Geometry: final body of the model. Coordinates: model frame, mm. A direction names the side the tool comes from. Give positions to 0.01 mm unless a question says otherwise; leave off trailing zeros. Order: outer loops, then holes, each group sorted by start corner. A loop starts at its lowest first (then second) coordinate and runs counter-clockwise, first axis right, second up. Notation, with made-up numbers: (64.25, 55.25) -> (104.25, 55.25) arc R13 ccw to (104.25, 61.25) -> close; hole circle Ø5 at (-35, 81). An arc over 180 degrees is marked (long way). One line per question, with ' | ' between items.
from build123d import *

# Parameters (mm, degrees)
F1_DEPTH = 6.35
F3_DEPTH = 1.27
F5_DEPTH = 18.542


with BuildPart() as f1:
    # F0 (on Top) → F1 (new body)
    with BuildSketch(Plane.XY):
        with BuildLine():
            Line((8.6645979291, 6.620054795), (2.0859979291, 6.620054795))
            ThreePointArc((2.0859979291, 6.620054795), (-1.2007758112, 5.2586285353), (-2.5622020709, 1.971854795))
            Line((-2.5622020709, 1.971854795), (-2.5622020709, -4.606745205))
            ThreePointArc((-2.5622020709, -4.606745205), (-1.2007758112, -7.8935189453), (2.0859979291, -9.254945205))
            Line((2.0859979291, -9.254945205), (8.6645979291, -9.254945205))
            ThreePointArc((8.6645979291, -9.254945205), (11.9513716694, -7.8935189453), (13.3127979291, -4.606745205))
            Line((13.3127979291, -4.606745205), (13.3127979291, 1.971854795))
            ThreePointArc((13.3127979291, 1.971854795), (11.9513716694, 5.2586285353), (8.6645979291, 6.620054795))
        make_face()
        with BuildLine():
            ThreePointArc((-0.0222020709, 1.971854795), (0.595275413, 3.4625773111), (2.0859979291, 4.080054795))
            Line((2.0859979291, 4.080054795), (8.6645979291, 4.080054795))
            ThreePointArc((8.6645979291, 4.080054795), (10.1553204452, 3.4625773111), (10.7727979291, 1.971854795))
            Line((10.7727979291, 1.971854795), (10.7727979291, -4.606745205))
            ThreePointArc((10.7727979291, -4.606745205), (10.1553204452, -6.0974677211), (8.6645979291, -6.714945205))
            Line((8.6645979291, -6.714945205), (2.0859979291, -6.714945205))
            ThreePointArc((2.0859979291, -6.714945205), (0.595275413, -6.0974677211), (-0.0222020709, -4.606745205))
            Line((-0.0222020709, -4.606745205), (-0.0222020709, 1.971854795))
        make_face(mode=Mode.SUBTRACT)
    extrude(amount=F1_DEPTH)

    # F2 (on face) → F3 (join)
    with BuildSketch(Plane.XY.offset(6.35)):
        with BuildLine():
            Line((8.6645979291, 6.620054795), (2.0859979291, 6.620054795))
            ThreePointArc((2.0859979291, 6.620054795), (-1.2007758112, 5.2586285353), (-2.5622020709, 1.971854795))
            Line((-2.5622020709, 1.971854795), (-2.5622020709, -4.606745205))
            ThreePointArc((-2.5622020709, -4.606745205), (-1.2007758112, -7.8935189453), (2.0859979291, -9.254945205))
            Line((2.0859979291, -9.254945205), (8.6645979291, -9.254945205))
            ThreePointArc((8.6645979291, -9.254945205), (11.9513716694, -7.8935189453), (13.3127979291, -4.606745205))
            Line((13.3127979291, -4.606745205), (13.3127979291, 1.971854795))
            ThreePointArc((13.3127979291, 1.971854795), (11.9513716694, 5.2586285353), (8.6645979291, 6.620054795))
        make_face()
        with BuildLine():
            Line((-0.0222020709, -4.606745205), (-0.0222020709, 1.971854795))
            ThreePointArc((-0.0222020709, 1.971854795), (0.595275413, 3.4625773111), (2.0859979291, 4.080054795))
            Line((2.0859979291, 4.080054795), (8.6645979291, 4.080054795))
            ThreePointArc((8.6645979291, 4.080054795), (10.1553204452, 3.4625773111), (10.7727979291, 1.971854795))
            Line((10.7727979291, 1.971854795), (10.7727979291, -4.606745205))
            ThreePointArc((10.7727979291, -4.606745205), (10.1553204452, -6.0974677211), (8.6645979291, -6.714945205))
            Line((8.6645979291, -6.714945205), (2.0859979291, -6.714945205))
            ThreePointArc((2.0859979291, -6.714945205), (0.595275413, -6.0974677211), (-0.0222020709, -4.606745205))
        make_face(mode=Mode.SUBTRACT)
        with BuildLine():
            ThreePointArc((2.0859979291, 4.080054795), (0.595275413, 3.4625773111), (-0.0222020709, 1.971854795))
            Line((-0.0222020709, 1.971854795), (-0.0222020709, -4.606745205))
            ThreePointArc((-0.0222020709, -4.606745205), (0.595275413, -6.0974677211), (2.0859979291, -6.714945205))
            Line((2.0859979291, -6.714945205), (8.6645979291, -6.714945205))
            ThreePointArc((8.6645979291, -6.714945205), (10.1553204452, -6.0974677211), (10.7727979291, -4.606745205))
            Line((10.7727979291, -4.606745205), (10.7727979291, 1.971854795))
            ThreePointArc((10.7727979291, 1.971854795), (10.1553204452, 3.4625773111), (8.6645979291, 4.080054795))
            Line((8.6645979291, 4.080054795), (2.0859979291, 4.080054795))
        make_face()
        with BuildLine():
            Line((2.0859979291, 6.620054795), (-2.5622020709, 6.620054795))
            Line((-2.5622020709, 6.620054795), (-2.5622020709, 1.971854795))
            ThreePointArc((-2.5622020709, 1.971854795), (-1.2007758112, 5.2586285353), (2.0859979291, 6.620054795))
        make_face()
        with BuildLine():
            ThreePointArc((2.0859979291, -9.254945205), (-1.2007758112, -7.8935189453), (-2.5622020709, -4.606745205))
            Line((-2.5622020709, -4.606745205), (-2.5622020709, -9.254945205))
            Line((-2.5622020709, -9.254945205), (2.0859979291, -9.254945205))
        make_face()
        with BuildLine():
            Line((13.3127979291, -9.254945205), (13.3127979291, -4.606745205))
            ThreePointArc((13.3127979291, -4.606745205), (11.9513716694, -7.8935189453), (8.6645979291, -9.254945205))
            Line((8.6645979291, -9.254945205), (13.3127979291, -9.254945205))
        make_face()
        with BuildLine():
            Line((13.3127979291, 6.620054795), (8.6645979291, 6.620054795))
            ThreePointArc((8.6645979291, 6.620054795), (11.9513716694, 5.2586285353), (13.3127979291, 1.971854795))
            Line((13.3127979291, 1.971854795), (13.3127979291, 6.620054795))
        make_face()
    extrude(amount=F3_DEPTH)

    # F4 (on face) → F5 (join)
    with BuildSketch(Plane.XY.offset(7.62)):
        Polygon((3.3965749548, 2.0775151044), (1.4346468435, -1.3400371025), (3.4133698178, -4.7478927907), (7.3540209034, -4.7381962721), (9.3159490147, -1.3206440652), (7.3372260404, 2.0872116231), align=None)
    extrude(amount=F5_DEPTH)


solid = f1.part
1) Material intervals for probe 1 along Y at (x, z) = (3.5, 5.5); probe 2 along Z at (x, y) = (4.5, -3); probe 3 along Z at (x, y) = (7, 5.5), sorted ascending. Write a range as from..to.
Check result:
probe 1: y = -9.25..-6.71, 4.08..6.62 | probe 2: z = 6.35..26.16 | probe 3: z = 0..7.62
2) Section B-B on y = -7.5. Return loops of the section in (x, z).
Check result:
outline: (-2.56, 6.35) -> (-1.55, 6.35) -> (-1.55, 0) -> (12.3, 0) -> (12.3, 6.35) -> (13.31, 6.35) -> (13.31, 7.62) -> (-2.56, 7.62) -> close
3) Contact query for flat-ended pins moving along their axis: pin 1 Ø3 at (x, y) = (8, 0) entering from -Z; pin 2 Ø4 at (y, z) = (0, 15.5) entering from +X; pin 3 Ø1.5 at (x, z) = (10, 15) entering from +Y. Output: stop coordinate, or through.
Check result:
pin 1: stops at z = 6.35 | pin 2: stops at x = 9.32 | pin 3: stops at y = -1.21
4) Section A-A on z = 12.25. Return loops of the section in (x, y), plus the area to 3 significant figures.
Check result:
outline: (1.43, -1.34) -> (3.41, -4.75) -> (7.35, -4.74) -> (9.32, -1.32) -> (7.34, 2.09) -> (3.4, 2.08) -> close | area: 40.3 mm^2
5) Section C-C on x = -0.5. Return loops of the section in (y, z), plus the area to 3 significant figures.
Check result:
outline: (-9.25, 6.35) -> (-8.47, 6.35) -> (-8.47, 0) -> (5.83, 0) -> (5.83, 6.35) -> (6.62, 6.35) -> (6.62, 7.62) -> (-9.25, 7.62) -> close | area: 111 mm^2
6) Set-up query: faces 1 (the flat face through (-2, 6, 6.35)), 2 (the flat face through (8.34, 0.36, 16.76)), 3 (the flat face through (10.773, -1, 3)), 4 (the flat face through (12.4, -8.3, 6.35)), 5 (the flat face through (2.4, -3, 16.8)). Return all of +Z, -Z, +X, -X, +Y, -Y with unobstructed straight access to the full face (end or side cutting, diameter ignored); none if empty.
Check result:
face 1: -Z, -X, +Y | face 2: +Z, +X, +Y | face 3: -Z | face 4: -Z, +X, -Y | face 5: +Z, -X, -Y
7) Section D-D on y = 0.5. Return loops of the section in (x, z), plus the area to 3 significant figures.
Check result:
outline: (-2.56, 0) -> (-0.02, 0) -> (-0.02, 6.35) -> (10.77, 6.35) -> (10.77, 0) -> (13.31, 0) -> (13.31, 7.62) -> (8.26, 7.62) -> (8.26, 26.16) -> (2.49, 26.16) -> (2.49, 7.62) -> (-2.56, 7.62) -> close | area: 159 mm^2
8) Pull-direction query (Y, two-part tool) for faces 6 (the flat face through (-2.562, -1, 5)), 7 (the cylindrical face through (0.6, -6.1, 3.1)), 8 (the flat face through (8.321, -3.053, 16.761)), 9 (the flat face through (5, 4.08, 3)); classes: +Y half, -Y half, draft (parallel to the pull), parting line (faces both ways), or undercut.
Check result:
face 6: draft | face 7: undercut | face 8: -Y half | face 9: undercut
